Source: CAD feature listing. Evaluate the final solid. Frame: model axes, mm. A direction names the side the tool comes from. Round coordinates to 2 decimals unless told otherwise and drop trailing zeros. Loops run counter-clockwise (first coordinate to the right, second up) from the corner with the lowest first, then second, coordinate; pieces in that order, holes last. Notation, with made-up numbers: M 49,71 L 79,71 A24 cw 79,107 Z; hole C 26.25,8 d11. An arc over 180 degrees is marked long. Answer as a JSON object with one key per item and string values.
from build123d import *

# Parameters (mm, degrees)
F0_R     = 11.5
F1_DEPTH = 1
F2_R     = 12.25
F3_DEPTH = 3.5
F4_R     = 10.75
F5_DEPTH = 2.5
F6_R     = 0.508
F7_R     = 2.5
F7_R_2   = 1.5
F8_DEPTH = 2


with BuildPart() as f1:
    # F0 (on Top) → F1 (new body)
    with BuildSketch(Plane.XY):
        Circle(F0_R)
    extrude(amount=F1_DEPTH)

    # F2 (on face) → F3 (join)
    with BuildSketch(Plane.XY.offset(1)):
        Circle(F2_R)
    extrude(amount=F3_DEPTH)

    # F4 (on face) → F5 (cut)
    with BuildSketch(Plane.XY.offset(4.5)):
        Circle(F4_R)
    extrude(amount=-F5_DEPTH, mode=Mode.SUBTRACT)

    # F6
    f6_edges = [f1.edges().sort_by_distance(p)[0] for p in [
        (-12.25, 0, 1),
    ]]
    fillet(f6_edges, radius=F6_R)

    # F7 (on face) → F8 (join)
    with BuildSketch(Plane.XY.offset(2)):
        with Locations((-7.1, 0)):
            Circle(F7_R)
        with Locations((-7.1, 0)):
            Circle(F7_R_2, mode=Mode.SUBTRACT)
        with Locations((7.1, 0)):
            Circle(F7_R)
        with Locations((7.1, 0)):
            Circle(F7_R_2, mode=Mode.SUBTRACT)
    extrude(amount=F8_DEPTH)


solid = f1.part
Item 1: Section B-B on x = 0. Return the cut outline in (y, z).
Answer sheet:
{"outline": "M -12.25,1.51 A0.51 ccw -11.74,1 L -11.5,1 L -11.5,0 L 11.5,0 L 11.5,1 L 11.74,1 A0.51 ccw 12.25,1.51 L 12.25,4.5 L 10.75,4.5 L 10.75,2 L -10.75,2 L -10.75,4.5 L -12.25,4.5 Z"}
Item 2: Contact query for flat-ended pins moving along their axis: pin 1 Ø1.5 at (x, y) = (7, -1) entering from +Z; pin 2 Ø2 at (x, z) = (-2, 3) entering from -Y; pin 3 Ø0.9 at (x, y) = (-6.5, 0) entering from +Z. Output: stop coordinate, or through.
Answer sheet:
{"pin 1": "stops at z = 4", "pin 2": "stops at y = -12.21", "pin 3": "stops at z = 2"}
Item 3: Pull-direction query (Y, two-part tool) for faces 4 (the flat face through (0, -11, 4.5)), 5 (the cylindrical face through (6.586, 10.329, 2.983)), 6 (the flat face through (0, 0, 2)), 7 (the flat face through (7, -2, 4)); classes: pulls with the +Y half, pulls with the -Y half, needs draft (parallel to the pull), parting line crosses it, or undercut.
Answer sheet:
{"face 4": "needs draft", "face 5": "parting line crosses it", "face 6": "undercut", "face 7": "undercut"}
Item 4: Section A-A on z = 2.95. Return the cut outline in (x, y).
Answer sheet:
{"outline": "C 0,0 d24.5; C -7.1,0 d5; C 7.1,0 d5; hole C 0,0 d21.5; hole C -7.1,0 d3; hole C 7.1,0 d3"}
Item 5: Access query for faces 1 (the flat face through (0, 0, 0)), 2 (the cylindrical face through (-1.5, 11.4, 0.5)), 3 (the cylindrical face through (-5.714, -0.575, 2.986)). Directions: +Z, -Z, +X, -X, +Y, -Y. A direction counts if a zero-diameter tool reaches every point of the face in a straight line with its end or side. Return the directions, or none.
Answer sheet:
{"face 1": "-Z, +X, -X, +Y, -Y", "face 2": "-Z", "face 3": "+Z"}
Item 6: Line query: probe 1 along Y at (x, z) = (-7.1, 3.2); probe 2 along Y at (x, z) = (0.25, 3.15); probe 3 along Y at (x, z) = (-8, 3.75). Output: solid intervals per line, ascending. Write a range as from..to.
Answer sheet:
{"probe 1": "y = -9.98..-8.07, -2.5..-1.5, 1.5..2.5, 8.07..9.98", "probe 2": "y = -12.25..-10.75, 10.75..12.25", "probe 3": "y = -9.28..-7.18, -2.33..-1.2, 1.2..2.33, 7.18..9.28"}
